Design review of the part shown in the three views and the two pictorial views. Dimensions are in mm from the part's minimum x, y and z. A direction names the side the tool comes from. Round coordinates to 2 decimals unless told otherwise and drop trailing zeros. Write each loop counter-clockwise with the first axis right and the second up, starting at its lowest first coordinate (ties: lowest second). Pieces come first, ordered by that corner, then holes. Notation, with made-up numbers: (1.25, 68.5) -> (25.25, 68.5) arc R13 cw to (25.25, 86.5) -> close; hole circle Ø4 at (48.5, 55). An arc over 180 degrees is marked (long way). One line per question, with ' | ' between items. Start each with the question number.
1) Insertion check: pin 1 Ø14 at (x, y) = (4, 46) entering from -Z; pin 2 Ø5 at (y, z) = (53, 9) entering from -X; pin 3 Ø4 at (y, z) = (43, 7) entering from +X. Each pin has a flat end and moves straight along its axis. Give the tip position at first contact, or say it passes through.
2) For probe 1 along Z at (x, y) = (49, 53.5) (1 decimal); probe 2 along Y at (x, z) = (17.5, 3.5); probe 3 along X at (y, z) = (44, 3.75), list the stretches that pass through material, from the lowest coordinate up.
3) Mouldability with a two-part tool opening along X and no side actions: class the marked faces 4, 5 and 6 as +X half, -X half, draft (parallel to the pull), parting line (faces both ways), or undercut.
4) Consider section A-A (y = 61). Give the boundary of the cut face in (x, z) (1 decimal), then the cut area to 3 significant figures.
5) Consider section C-C (x = 11). Give the boundary of the cut face in (y, z) (1 decimal), then the cut area to 3 significant figures.
6) For the marked faces 1, 2 and 3, list the 3-axis set-ups (+Z, -Z, +X, -X, +Y, -Y) from which the entire face can be reached by the end or side of a thin tool; tool diameter is ignored.
7) Consider section B-B (z = 10.75). Give the boundary of the cut face in (x, y).
8) Consider section D-D (y = 16). Give the boundary of the cut face in (x, z) (1 decimal).
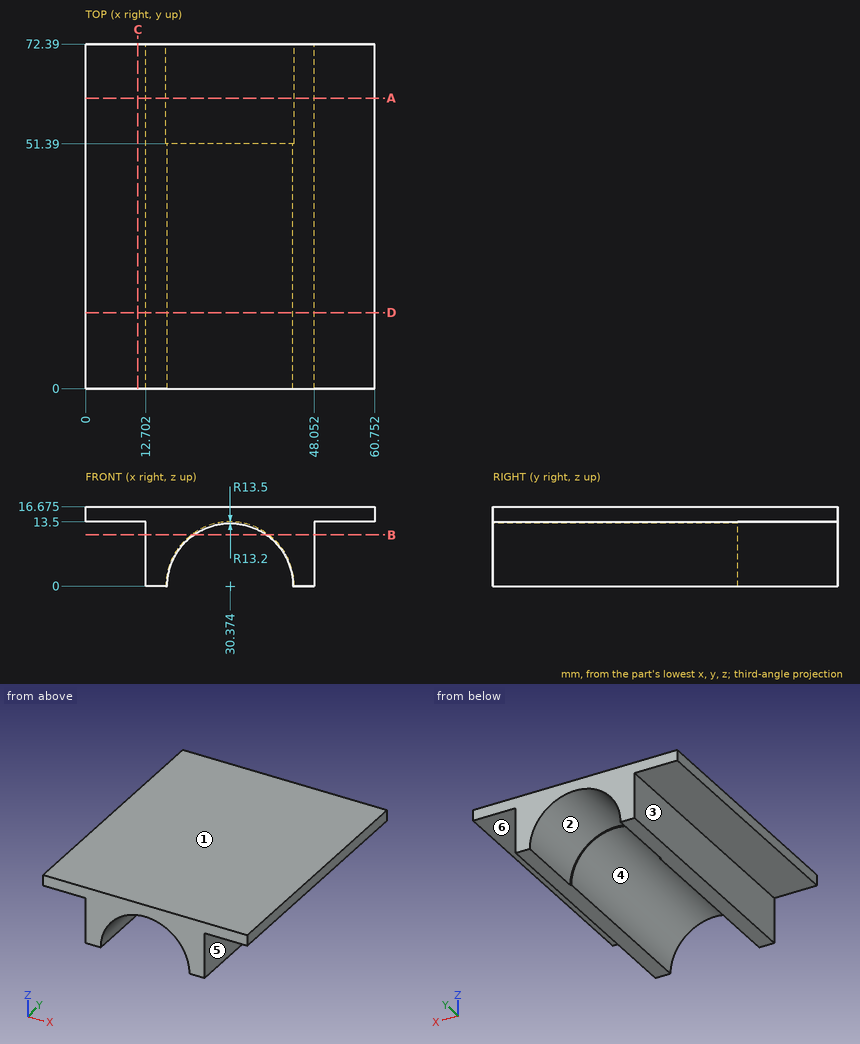
From the geometry:
1) pin 1: stops at z = 13.5 | pin 2: stops at x = 12.7 | pin 3: stops at x = 48.05
2) probe 1: z = 13.5 to 16.7 | probe 2: y = 0 to 51.39 | probe 3: x = 12.7 to 17.72, 43.03 to 48.05
3) face 4: undercut | face 5: +X half | face 6: draft
4) outline: (0, 13.5) -> (12.7, 13.5) -> (12.7, 0) -> (16.9, 0) arc R13.5 cw to (43.9, 0) -> (48.1, 0) -> (48.1, 13.5) -> (60.8, 13.5) -> (60.8, 16.7) -> (0, 16.7) -> close | area: 384 mm2
5) outline: (0, 13.5) -> (72.4, 13.5) -> (72.4, 16.7) -> (0, 16.7) -> close | area: 230 mm2
6) face 1: +Z, +X, -X, +Y, -Y | face 2: -Z, +Y | face 3: -Z, -X, +Y, -Y
7) outline: (12.7, 0) -> (22.71, 0) -> (22.71, 51.39) -> (22.21, 51.39) -> (22.21, 72.39) -> (12.7, 72.39) -> close; (38.03, 0) -> (48.05, 0) -> (48.05, 72.39) -> (38.54, 72.39) -> (38.54, 51.39) -> (38.03, 51.39) -> close
8) outline: (0, 13.5) -> (12.7, 13.5) -> (12.7, 0) -> (17.2, 0) arc R13.2 cw to (43.6, 0) -> (48.1, 0) -> (48.1, 13.5) -> (60.8, 13.5) -> (60.8, 16.7) -> (0, 16.7) -> close
